Study the drawing (mm; zero at the part's minimum x, y, z) and answer. A direction names the side the tool comes from. Coordinates: 2 decimals unless noted, no trailing zeros. Order: outer loops, then holes, each group sorted by start corner. A loop starts at its lowest first (then second) coordinate and runs counter-clockwise, first axis right, second up. Notation, with made-up numbers: (62, 89) -> (106, 89) arc R26 ccw to (106, 127) -> close; hole circle Ø9 at (-30, 69.25). An arc over 180 degrees is marked (long way). One line per question, with ' | ' between items.
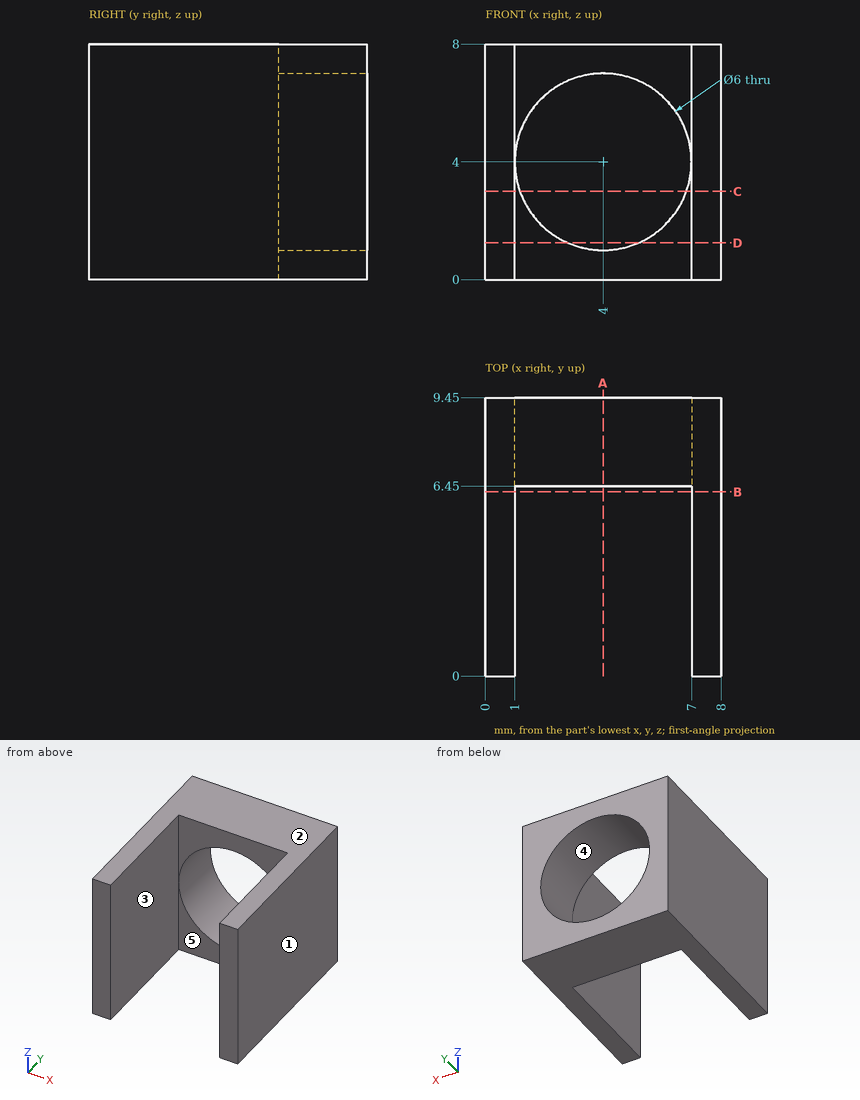
Item 1: Each of these flat-tipped pins is pushed along its axis until it touches: pin 1 Ø3 at (x, y) = (3, 3.5) entering from +Z; pin 2 Ø2 at (x, z) = (4.5, 2) entering from -Y. Where does it stop, or does it pass through?
Computed values:
pin 1: passes through | pin 2: stops at y = 6.45
Item 2: Section A-A, the plane x = 4 is taken. Give the vertices of the cut face in (y, z), plus the area to 3 significant figures.
Computed values:
outline: (6.45, 0) -> (9.45, 0) -> (9.45, 1) -> (6.45, 1) -> close; (6.45, 7) -> (9.45, 7) -> (9.45, 8) -> (6.45, 8) -> close | area: 6.00 mm^2
Item 3: Section C-C, the plane z = 3 is taken. Give the vertices of the cut face in (x, y), plus the area to 3 significant figures.
Computed values:
outline: (0, 0) -> (1, 0) -> (1, 6.45) -> (1.17, 6.45) -> (1.17, 9.45) -> (0, 9.45) -> close; (6.83, 6.45) -> (7, 6.45) -> (7, 0) -> (8, 0) -> (8, 9.45) -> (6.83, 9.45) -> close | area: 19.9 mm^2
Item 4: Determine the mould class of the marked faces 1, 2 and 3 for opening direction X: pulls with the +X half, pulls with the -X half, needs draft (parallel to the pull), parting line crosses it, or undercut.
Computed values:
face 1: pulls with the +X half | face 2: needs draft | face 3: undercut
Item 5: Find the intervals of material crossed by L1, parallel to X at y = 5.75, z = 3.5; L2, parallel to Y at x = 5, z = 0.5, in increasing order.
Computed values:
L1: x = 0 to 1, 7 to 8 | L2: y = 6.45 to 9.45
Item 6: Section B-B, the plane y = 6.25 is taken. Give the vertices of the cut face in (x, z).
Computed values:
outline: (0, 0) -> (1, 0) -> (1, 8) -> (0, 8) -> close; (7, 0) -> (8, 0) -> (8, 8) -> (7, 8) -> close
Item 7: Section D-D, the plane z = 1.25 is taken. Give the vertices of the cut face in (x, y).
Computed values:
outline: (0, 0) -> (1, 0) -> (1, 6.45) -> (2.8, 6.45) -> (2.8, 9.45) -> (0, 9.45) -> close; (5.2, 6.45) -> (7, 6.45) -> (7, 0) -> (8, 0) -> (8, 9.45) -> (5.2, 9.45) -> close
Item 8: For the marked faces 4 and 5, determine the directions among +Z, -Z, +X, -X, +Y, -Y from which every point of the face is accessible in a straight line to the end or side of a thin tool.
Computed values:
face 4: +Y, -Y | face 5: +Z, -Z, -Y
